Input: part model. Units: mm. Frame: model coordinates. Face numbers are marked on the shaded views. A direction names the side the tool comes from. Round coordinates to 2 decimals unless told otherwise and drop trailing zeros. Loops run counter-clockwise (first coordinate to the right, second up) from the corner with the lowest first, then second, coordinate; pieces in that order, holes last. Notation, with made-up numbers: (65, -40) -> (114, -40) arc R5 cw to (114, -32) -> close; hole circle Ø10 at (23, 5). An arc over 180 degrees is marked (long way). Answer as a JSON object with one key per item and string values.
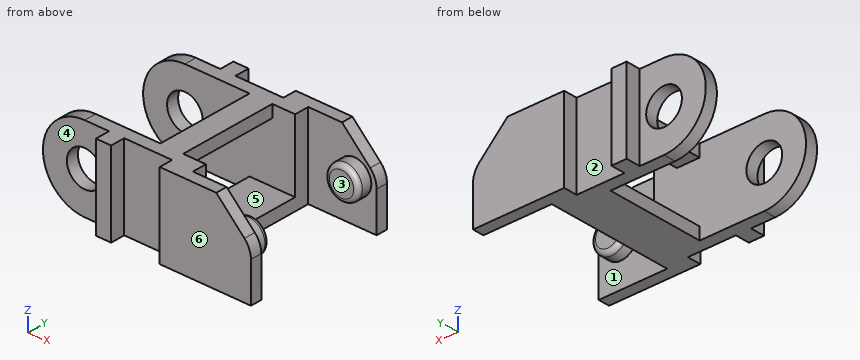
```python
from build123d import *

# Parameters (mm, degrees)
SKETCH_R        = 2.35
PAD_DEPTH       = 16.22
PAD001_DEPTH    = 19.84
SKETCH010_W     = 14
SKETCH010_H     = 13
POCKET_DEPTH    = 1.611
POCKET001_DEPTH = 7.78
SKETCH012_W     = 14
SKETCH012_H     = 13
POCKET002_DEPTH = 1.61
SKETCH013_W     = 2
SKETCH013_H     = 1.91
PAD002_DEPTH    = 11
SKETCH014_R     = 2.2
PAD003_DEPTH    = 1.91
SKETCH015_R     = 2.2
PAD004_DEPTH    = 1.91
FILLET_R        = 0.6


with BuildPart() as part:
    # Sketch → Pad (new body)
    with BuildSketch(Plane.XZ):
        with BuildLine():
            Line((20, 0), (20, 11))
            Line((20, 11), (5.500002, 11))
            ThreePointArc((5.500002, 11), (0, 5.5), (5.500002, 0))
            Line((20, 0), (5.500002, 0))
        make_face()
        with Locations((5.5, 5.5)):
            Circle(SKETCH_R, mode=Mode.SUBTRACT)
    extrude(amount=PAD_DEPTH)

    # Sketch009 → Pad001 (join)
    with BuildSketch(Plane.XZ.offset(-1.81)):
        with BuildLine():
            Line((17, 0), (29, 0))
            Line((29, 0), (29, 5.242431))
            ThreePointArc((29, 5.242431), (28.779251, 6.352213), (28.15061, 7.293041))
            Line((24.443651, 11), (28.15061, 7.293041))
            Line((17, 11), (24.443651, 11))
            Line((17, 11), (17, 0))
        make_face()
    extrude(amount=PAD001_DEPTH)

    # Sketch010 → Pocket (cut, through all)
    with BuildSketch(Plane.XY.offset(1.61)):
        Polygon((20, -1.61), (20, -14.61), (20, -16.52), (29, -16.52), (29, 0.3), (20, 0.3), align=None)
        with Locations((7, -8.11)):
            Rectangle(SKETCH010_W, SKETCH010_H)
    extrude(amount=-POCKET_DEPTH, mode=Mode.SUBTRACT)

    # Sketch011 → Pocket001 (cut)
    with BuildSketch(Plane.XY.offset(9.39)):
        Polygon((0, -14.61), (0, -1.61), (14, -1.61), (20, -1.61), (20, 0.3), (29, 0.3), (29, -16.52), (20, -16.52), (20, -14.61), (14, -14.61), align=None)
    extrude(amount=-POCKET001_DEPTH, mode=Mode.SUBTRACT)

    # Sketch012 → Pocket002 (cut)
    with BuildSketch(Plane.XY.offset(11)):
        with Locations((7, -8.11)):
            Rectangle(SKETCH012_W, SKETCH012_H)
        Polygon((20, 0.3), (29, 0.3), (29, -16.52), (20, -16.52), (20, -14.61), (17, -14.61), (17, -1.61), (20, -1.61), align=None)
    extrude(amount=-POCKET002_DEPTH, mode=Mode.SUBTRACT)

    # Sketch013 → Pad002 (join)
    with BuildSketch(Plane.XY):
        with Locations((9.7, 0.955)):
            Rectangle(SKETCH013_W, SKETCH013_H)
        with Locations((9.7, -17.175)):
            Rectangle(SKETCH013_W, SKETCH013_H)
    extrude(amount=PAD002_DEPTH)

    # Sketch014 → Pad003 (join)
    with BuildSketch(Plane.XZ.offset(-0.3)):
        with Locations((26.1, 5.5)):
            Circle(SKETCH014_R)
    extrude(amount=PAD003_DEPTH)

    # Sketch015 → Pad004 (join)
    with BuildSketch(Plane.XZ.offset(16.52)):
        with Locations((26.1, 5.5)):
            Circle(SKETCH015_R)
    extrude(amount=-PAD004_DEPTH)

    # Fillet
    fillet_edges = [part.edges().sort_by_distance(p)[0] for p in [
        (23.9, -1.61, 5.5),
        (23.9, -14.61, 5.5),
    ]]
    fillet(fillet_edges, radius=FILLET_R)


solid = part.part
```
1) Ray query, probe 1 along Y at (x, z) = (3, 1.5); probe 2 along Y at (x, z) = (24, 2.25); probe 3 along X at (y, z) = (-2.25, 10). Return the intervals inside material, ascending.
Output:
{"probe 1": "y = -16.22 to -14.61, -1.61 to 0", "probe 2": "y = -18.03 to -16.52, 0.3 to 1.81", "probe 3": "x = 14 to 17"}
2) Section B-B, the plane x = 14.5. Output: boundary loops of the cut face in (y, z), plus the area to 3 significant figures.
Output:
{"outline": "(-16.22, 0) -> (0, 0) -> (0, 11) -> (-16.22, 11) -> close; hole (-14.61, 1.61) -> (-1.61, 1.61) -> (-1.61, 9.39) -> (-14.61, 9.39) -> close", "area": "77.3 mm^2"}
3) Section A-A, the plane y = -3.75. Output: boundary loops of the cut face in (x, z).
Output:
{"outline": "(14, 0) -> (20, 0) -> (20, 1.61) -> (14, 1.61) -> close; (14, 9.39) -> (17, 9.39) -> (17, 11) -> (14, 11) -> close"}
4) Section D-D, the plane z = 2. Output: boundary loops of the cut face in (x, y), plus the area to 3 significant figures.
Output:
{"outline": "(1.26, -16.22) -> (8.7, -16.22) -> (8.7, -18.13) -> (10.7, -18.13) -> (10.7, -16.22) -> (17, -16.22) -> (17, -18.03) -> (29, -18.03) -> (29, -16.52) -> (20, -16.52) -> (20, -14.61) -> (1.26, -14.61) -> close; (1.26, -1.61) -> (20, -1.61) -> (20, 0.3) -> (29, 0.3) -> (29, 1.81) -> (17, 1.81) -> (17, 0) -> (10.7, 0) -> (10.7, 1.91) -> (8.7, 1.91) -> (8.7, 0) -> (1.26, 0) -> close", "area": "106 mm^2"}
5) Reachability of the marked faces 4, 5 and 6 from +Z, -Z, +X, -X, +Y, -Y: full face, straight path, thin tool, end or side. Return the list, or none.
Output:
{"face 4": "+Z, -Z, -X, -Y", "face 5": "+X, -X", "face 6": "+Z, -Z, +X, -Y"}
6) Draft query along X for the marked faces 1, 2 and 3. Return one class per face: +X half, -X half, draft (parallel to the pull), parting line (faces both ways), or undercut.
Output:
{"face 1": "undercut", "face 2": "undercut", "face 3": "draft"}
7) Section C-C, the plane x = 3.5. Output: boundary loops of the cut face in (y, z).
Output:
{"outline": "(-16.22, 0.38) -> (-14.61, 0.38) -> (-14.61, 4.27) -> (-16.22, 4.27) -> close; (-16.22, 6.73) -> (-14.61, 6.73) -> (-14.61, 10.62) -> (-16.22, 10.62) -> close; (-1.61, 0.38) -> (0, 0.38) -> (0, 4.27) -> (-1.61, 4.27) -> close; (-1.61, 6.73) -> (0, 6.73) -> (0, 10.62) -> (-1.61, 10.62) -> close"}
8) Contact query for flat-ended pins moving along their axis: P1, Ø6, axis at y = -3.5, z = 5.5, coming from the +X side; P2, Ø4, axis at x = 5.5, z = 5.5, coming from the -Y side; P3, Ø0.5, axis at y = -11.5, z = 0.5, coming from the -X side; P4, Ø4, axis at x = 16.5, z = 7.5, coming from the -Y side. Output: stop coordinate, or through.
Output:
{"P1": "stops at x = 28.3", "P2": "passes through", "P3": "stops at x = 14", "P4": "stops at y = -18.03"}
